The model under review builds one solid part; all positions refer to its coordinate system, in mm. A direction names the side the tool comes from. Round coordinates to 2 decimals unless told otherwise and drop trailing zeros. Write each loop counter-clockwise with the first axis right and the second up, starting at its lowest first coordinate (ties: lowest second). Pieces come first, ordered by that corner, then holes. Notation, with made-up numbers: (-4, 56) - (50, 56) arc R16 cw to (50, 70) - close; hole circle Ø3 at (6.25, 40.5). An arc over 180 degrees is marked (long way). Return JSON: item names as keys, results as strings.
from build123d import *

# Parameters (mm, degrees)
SKETCH1_R           = 15.07617
BOSS_EXTRUDE1_DEPTH = 24.9071592
SKETCH2_R           = 9.3853
SKETCH2_R_2         = 4.5847
BOSS_EXTRUDE2_DEPTH = 4.7498
SKETCH3_R           = 7.5
CUT_EXTRUDE1_DEPTH  = 18.75
BOSS_EXTRUDE3_START = 20
SKETCH4_R           = 11
SKETCH4_R_2         = 7.5
BOSS_EXTRUDE3_DEPTH = 20
CUT_EXTRUDE4_START  = -8.3023864
SKETCH5_R           = 15.07617
SKETCH5_R_2         = 10
CUT_EXTRUDE4_DEPTH  = 8.3023864


with BuildPart() as part:
    # Sketch1 → Boss-Extrude1 (new body)
    with BuildSketch(Plane(origin=(0, 0, 0), x_dir=(0, 0, -1), z_dir=(1, 0, 0))):
        with Locations(Location((0, 0, 0), (0, 0, 180))):
            Circle(SKETCH1_R)
    extrude(amount=BOSS_EXTRUDE1_DEPTH)

    # Sketch2 → Boss-Extrude2 (add)
    with BuildSketch(Plane.ZY):
        with Locations(Location((0, 0, 0), (0, 0, 180))):
            Circle(SKETCH2_R)
        Circle(SKETCH2_R_2, mode=Mode.SUBTRACT)
    extrude(amount=BOSS_EXTRUDE2_DEPTH)

    # Sketch3 → Cut-Extrude1 (cut)
    with BuildSketch(Plane(origin=(24.9071592, 0, 0), x_dir=(0, 0, -1), z_dir=(1, 0, 0))):
        Circle(SKETCH3_R)
    extrude(amount=-CUT_EXTRUDE1_DEPTH, mode=Mode.SUBTRACT)

    # Sketch4 → Boss-Extrude3 (add)
    with BuildSketch(Plane(origin=(24.9071592, 0, 0), x_dir=(0, 0, -1), z_dir=(1, 0, 0)).offset(BOSS_EXTRUDE3_START)):
        Circle(SKETCH4_R)
        Circle(SKETCH4_R_2, mode=Mode.SUBTRACT)
    extrude(amount=-BOSS_EXTRUDE3_DEPTH)

    # Sketch5 → Cut-Extrude4 (cut)
    with BuildSketch(Plane(origin=(16.6047728, 0, 0), x_dir=(0, 0, -1), z_dir=(1, 0, 0)).offset(CUT_EXTRUDE4_START)):
        with Locations(Location((0, 0, 0), (0, 0, 180))):
            Circle(SKETCH5_R)
        Circle(SKETCH5_R_2, mode=Mode.SUBTRACT)
    extrude(amount=CUT_EXTRUDE4_DEPTH, mode=Mode.SUBTRACT)


solid = part.part
(1) Add section D-D (y = -13). Write out the cut boundary in (x, z), plus the area to 3 significant figures.
Filled in:
{"outline": "(0, -7.63) - (8.3, -7.63) - (8.3, 7.63) - (0, 7.63) - close; (16.6, -7.63) - (24.91, -7.63) - (24.91, 7.63) - (16.6, 7.63) - close", "area": "254 mm2"}
(2) Add section B-B (y = 1.5). Write out the cut boundary in (x, z).
Filled in:
{"outline": "(-4.75, -9.26) - (0, -9.26) - (0, -15) - (8.3, -15) - (8.3, -9.89) - (16.6, -9.89) - (16.6, -15) - (24.91, -15) - (24.91, -10.9) - (44.91, -10.9) - (44.91, -7.35) - (6.16, -7.35) - (6.16, 7.35) - (44.91, 7.35) - (44.91, 10.9) - (24.91, 10.9) - (24.91, 15) - (16.6, 15) - (16.6, 9.89) - (8.3, 9.89) - (8.3, 15) - (0, 15) - (0, 9.26) - (-4.75, 9.26) - (-4.75, 4.33) - (0, 4.33) - (0, -4.33) - (-4.75, -4.33) - close"}
(3) Clearance check with flat-ended pins moving along their axes: pin 1 Ø1.5 at (x, y) = (18.5, -12) entering from -Z; pin 2 Ø12 at (x, z) = (38.5, 10.5) entering from -Y; pin 3 Ø7.5 at (y, z) = (0, 0) entering from -X. State where each tip first meets the part, or that it passes through.
Filled in:
{"pin 1": "stops at z = -10.04", "pin 2": "stops at y = -10.04", "pin 3": "stops at x = 0"}
(4) Wall thickness on line 1 (X direction, y = -11, z = 4); line 2 (Y direction, x = 33, z = 0); line 3 (Y direction, x = 20, z = 0): over which ranges is each line inside the solid? List them lowest first.
Filled in:
{"line 1": "x = 0 to 8.3, 16.6 to 24.91", "line 2": "y = -11 to -7.5, 7.5 to 11", "line 3": "y = -15.08 to -7.5, 7.5 to 15.08"}
(5) For faces 1 (the flat face through (-4.75, 2, 4.3)), 2 (the cylindrical face through (-2.34, -2.79, -3.64)), 3 (the flat face through (6.157, 0, 0)), 4 (the cylindrical face through (12.4, -9.76, 2.17)), list the 3-axis set-ups (+Z, -Z, +X, -X, +Y, -Y) from which the entire face can be reached by the end or side of a thin tool; tool diameter is ignored.
Filled in:
{"face 1": "+Z, -Z, -X, +Y, -Y", "face 2": "-X", "face 3": "+X", "face 4": "none"}
(6) Mouldability with a two-part tool opening along X and no side actions: class faces 5 (the cylindrical face through (25.803, 0.33, 7.493)), 6 (the flat face through (16.605, 3, 10)), 7 (the flat face through (44.907, 2.6, -7.2)) as released by +X, released by -X, zero draft, split by the parting line, or undercut.
Filled in:
{"face 5": "zero draft", "face 6": "undercut", "face 7": "released by +X"}
(7) Add section C-C (x = 41.5). Write out the cut boundary in (y, z), plus the area to 3 significant figures.
Filled in:
{"outline": "circle Ø22 at (0, 0); hole circle Ø15 at (0, 0)", "area": "203 mm2"}
(8) Add section A-A (z = 0). Write out the cut boundary in (x, y).
Filled in:
{"outline": "(-4.75, -9.39) - (0, -9.39) - (0, -15.08) - (8.3, -15.08) - (8.3, -10) - (16.6, -10) - (16.6, -15.08) - (24.91, -15.08) - (24.91, -11) - (44.91, -11) - (44.91, -7.5) - (6.16, -7.5) - (6.16, 7.5) - (44.91, 7.5) - (44.91, 11) - (24.91, 11) - (24.91, 15.08) - (16.6, 15.08) - (16.6, 10) - (8.3, 10) - (8.3, 15.08) - (0, 15.08) - (0, 9.39) - (-4.75, 9.39) - (-4.75, 4.58) - (0, 4.58) - (0, -4.58) - (-4.75, -4.58) - close"}
